For this review, take the finished solid that the model builds, in its own axes (mm). Face numbers are marked on the shaded views. A direction names the side the tool comes from. Round coordinates to 2 decimals unless told otherwise and drop trailing zeros. Order: outer loops, then holes, each group sorted by start corner. A loop starts at its lowest first (then second) coordinate and runs counter-clockwise, first axis right, second up. Notation, with made-up numbers: (70, -29) - (91, -29) arc R29 ccw to (91, -7) - close; hole circle Ø8 at (83.25, 55). An arc over 180 degrees is marked (long way). One line per item, written item: value.
Autodesk Inventor part; units mm, degrees
ref_plane "bolt_XY" through (0, 0, 0) normal (1, 0, 0) x (0, 0, -1)
ref_plane "bolt_YZ" through (0, 0, 0) normal (0, 0, -1) x (0, 1, 0)
ref_plane "bolt_ZX" through (0, 0, 0) normal (0, 1, 0) x (1, 0, 0)
sketch "Sketch_1" plane through (0, 0, 0) normal (0, 0, 1) x (1, 0, 0)
  line L0 (25, 0) -> (-5, 0)
  line L1 (-5, 0) -> (-5, 4.25)
  line L2 (-5, 4.25) -> (0, 4.25)
  line L3 (0, 4.25) -> (0, 2.5)
  line L4 (0, 2.5) -> (24.5095, 2.5)
  line L5 (24.5095, 2.5) -> (25, 2.0095)
  line L6 (25, 2.0095) -> (25, 0)
  line L7 (25, 0) -> (-5, 0)
revolve "Revolution1" add sketch "Sketch_1" angle 360 about axis through (25, 0, 0) along (1, 0, 0)
thread "Thread1"
sketch "Sketch_4" plane through (0, 0, 0) normal (0, 0, 1) x (1, 0, 0)
  line L0 (-1.9641, 0) -> (-5, 0)
  line L1 (-5, 0) -> (-5, 2)
  line L2 (-5, 2) -> (-2.5, 2)
  line L3 (-2.5, 2) -> (-1.9641, 0)
  line L4 (-1.9641, 0) -> (-5, 0)
revolve "Revolution2" cut sketch "Sketch_4" angle 360 about axis through (-1.9641, 0, 0) along (1, 0, 0)
sketch "Sketch_3" plane through (-5, 0, 0) normal (1, 0, 0) x (0, 0, -1)
  line L0 (-2, 1.1547) -> (-2, -1.1547)
  line L1 (-2, -1.1547) -> (0, -2.3094)
  line L2 (0, -2.3094) -> (2, -1.1547)
  line L3 (2, -1.1547) -> (2, 1.1547)
  line L4 (2, 1.1547) -> (0, 2.3094)
  line L5 (0, 2.3094) -> (-2, 1.1547)
extrude "Extrusion1" cut sketch "Sketch_3" along normal blind 2.5
ref_plane "bolt_XY" through (0, 0, 0) normal (1, 0, 0) x (0, 0, -1)
ref_plane "bolt_YZ" through (0, 0, 0) normal (0, 0, -1) x (0, 1, 0)
ref_plane "bolt_ZX" through (0, 0, 0) normal (0, 1, 0) x (1, 0, 0)
ref_plane "nut_XY" through (25, 0, 0) normal (1, 0, 0) x (0, 0, -1)
ref_plane "nut_YZ" through (25, 0, 0) normal (0, 0, -1) x (0, 1, 0)
ref_plane "nut_ZX" through (25, 0, 0) normal (0, 1, 0) x (1, 0, 0)
properties part number "CBM5-25"
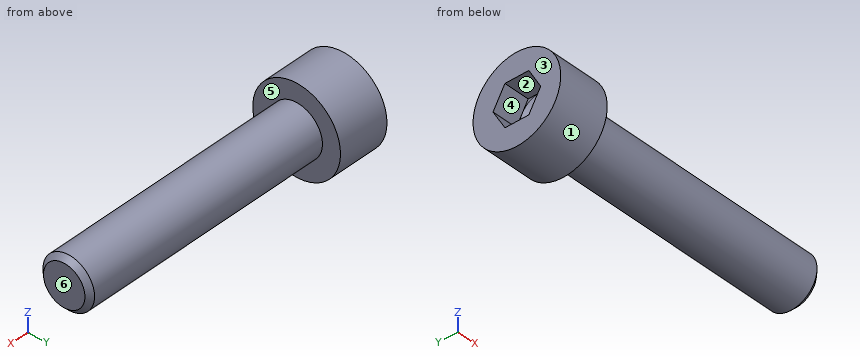
Item 1: For P1, Ø5, axis at x = -1.5, z = 2, coming from the -Y side; P2, Ø0.5, axis at y = 1, z = -1.5, coming from the -X side; P3, Ø1, axis at x = 7.5, z = 2, coming from the -Y side; P4, Ø3, axis at x = 17, y = 2.5, coming from the -Z side, all flat-tipped, find the tip position at first contact; note any pin that passes through.
Returned:
P1: y = -4.25
P2: x = -2.5
P3: y = -2
P4: z = -2.29
Item 2: Take a section at B-B (y = 3.75). Write out the cut boundary in (x, z), plus the area to 3 significant figures.
Returned:
outline: (-5, -2) - (0, -2) - (0, 2) - (-5, 2) - close
area: 20.0 mm^2
Item 3: Machinability: for the marked faces 4, 5 and 6, which of the approach directions +Z, -Z, +X, -X, +Y, -Y give a long, thin tool a straight path to every point of the face, cutting with its end or side? Answer none if there is none.
Returned:
face 4: -X
face 5: +X
face 6: +Z, -Z, +X, +Y, -Y
Item 4: Take a section at A-A (x = 0.5). Write out the cut boundary in (y, z).
Returned:
outline: circle Ø5 at (0, 0)
Item 5: Wall thickness on line 1 (Y direction, x = 23, z = -1.5); line 2 (X direction, y = 4, z = 1); line 3 (Z direction, x = -3.25, y = -2.25): over which ranges is each line inside the solid? List them lowest first.
Returned:
line 1: -2 to 2
line 2: -5 to 0
line 3: -3.61 to -0.1, 0.1 to 3.61
Item 6: The part is to be moulded in two halves that separate along Y. For the marked faces 1, 2 and 3, say which applies: +Y half, -Y half, draft (parallel to the pull), parting line (faces both ways), or undercut.
Returned:
face 1: parting line
face 2: undercut
face 3: draft
